Source: CAD feature listing. Evaluate the final solid. Frame: model axes, mm. Give positions to 0.01 mm unless a question says otherwise; leave off trailing zeros. Loops run counter-clockwise (first coordinate to the right, second up) from the corner with the lowest first, then second, coordinate; pieces in that order, holes last. Notation, with made-up numbers: (66.5, 61) -> (113.5, 61) arc R22 cw to (113.5, 95) -> close; hole circle Ø7 at (45, 23.5). An arc over 180 degrees is marked (long way). Put each result on its own line as item: value.
```python
from build123d import *

# Parameters (mm, degrees)
SZKIC2_W                    = 553
SZKIC2_H                    = 1.75
DODANIE_WYCI_GNI_CIE1_DEPTH = 290
WYTNIJ_WYCI_GNI_CIE1_DEPTH  = 10
SZKIC5_W                    = 548
SZKIC5_H                    = 1.75
DODANIE_WYCI_GNI_CIE2_DEPTH = 20


with BuildPart() as part:
    # Szkic2 → Dodanie-wyciągnięcie1 (new body)
    with BuildSketch(Plane.XY):
        with Locations((0, -0.875)):
            Rectangle(SZKIC2_W, SZKIC2_H)
    extrude(amount=DODANIE_WYCI_GNI_CIE1_DEPTH)

    # Szkic3 → Wytnij-wyciągnięcie1 (cut)
    with BuildSketch(Plane(origin=(0, 0, 0), x_dir=(1, 0, 0), z_dir=(0, 1, 0))):
        Polygon((276.5, -290), (146.5, -290), (276.5, -160), align=None)
    extrude(amount=-WYTNIJ_WYCI_GNI_CIE1_DEPTH, mode=Mode.SUBTRACT)

    # Szkic5 → Dodanie-wyciągnięcie2 (add)
    with BuildSketch(Plane.XZ.offset(1.75)):
        with Locations((-0.75, 0.875)):
            Rectangle(SZKIC5_W, SZKIC5_H)
    extrude(amount=DODANIE_WYCI_GNI_CIE2_DEPTH)


solid = part.part
```
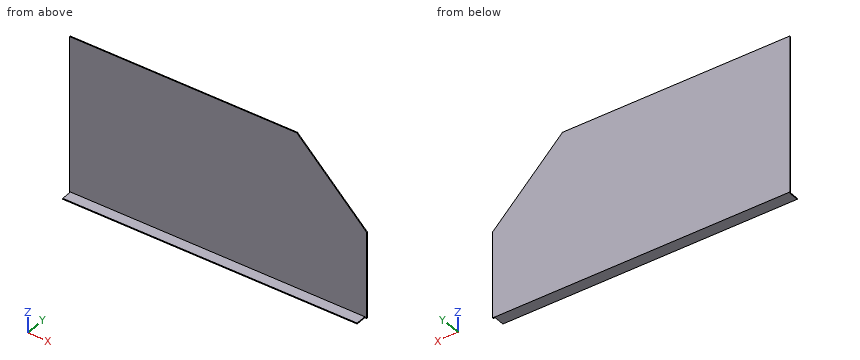
(1) First-contact query: P1, Ø8, axis at x = -68, z = 92.5, coming from the -Y side; P2, Ø12, axis at x = -169.5, y = -19, coming from the +Z side; P3, Ø0.9, axis at y = -10.5, z = 1, coming from the +X side. Flat tips, straight axial feed; report the tip coordinate or a pass-through.
Calculated:
P1: stops at y = -1.75
P2: stops at z = 1.75
P3: stops at x = 273.25
(2) Section C-C on y = -16. Return loops of the section in (x, z), then the cut area to 3 significant figures.
Calculated:
outline: (-274.75, 0) -> (273.25, 0) -> (273.25, 1.75) -> (-274.75, 1.75) -> close
area: 959 mm²
(3) Line query: probe 1 along Z at (x, y) = (-75, -3.75); probe 2 along Y at (x, z) = (-67, 34.5); probe 3 along X at (y, z) = (-1, 185.5). Output: solid intervals per line, ascending. Write a range as from..to.
Calculated:
probe 1: z = 0..1.75
probe 2: y = -1.75..0
probe 3: x = -276.5..251
(4) Section D-D on x = -58. Return loops of the section in (y, z), then the cut area to 4 significant figures.
Calculated:
outline: (-21.75, 0) -> (0, 0) -> (0, 290) -> (-1.75, 290) -> (-1.75, 1.75) -> (-21.75, 1.75) -> close
area: 542.5 mm²
(5) Section A-A on x = 223. Return loops of the section in (y, z), then the cut area to 3 significant figures.
Calculated:
outline: (-21.75, 0) -> (0, 0) -> (0, 213.5) -> (-1.75, 213.5) -> (-1.75, 1.75) -> (-21.75, 1.75) -> close
area: 409 mm²
(6) Section B-B on z = 201.5. Return loops of the section in (x, y), then the cut area to 3 significant figures.
Calculated:
outline: (-276.5, -1.75) -> (235, -1.75) -> (235, 0) -> (-276.5, 0) -> close
area: 895 mm²
